```python
from build123d import *

# Parameters (mm, degrees)
SKETCH1_R                = 13
SKETCH1_R_2              = 11
BOSS_EXTRUDE1_DEPTH      = 10
BOSS_EXTRUDE2_REACH      = 32.741
BOSS_EXTRUDE2_END_RADIUS = 13
SKETCH2_W                = 10
SKETCH2_H                = 26
SKETCH2_3_R              = 13
BOSS_EXTRUDE3_DEPTH      = 10


with BuildPart() as part:
    # Sketch1 → Boss-Extrude1 (new body)
    with BuildSketch(Plane(origin=(0, 0, 0), x_dir=(0, 0, -1), z_dir=(1, 0, 0))):
        Circle(SKETCH1_R)
        Circle(SKETCH1_R_2, mode=Mode.SUBTRACT)
    extrude(amount=BOSS_EXTRUDE1_DEPTH)

    # Boss-Extrude2: up to this cylinder (the profile starts outside it)
    boss_extrude2_end = Plane(origin=(5, 0, 0), z_dir=(-1, 0, 0)) * Cylinder(BOSS_EXTRUDE2_END_RADIUS, 92.482, mode=Mode.PRIVATE)
    # Sketch2 → Boss-Extrude2 (add, up to the surface)
    with BuildSketch(Plane(origin=(0, 13, 0), x_dir=(1, 0, 0), z_dir=(0, 1, 0)), mode=Mode.PRIVATE) as boss_extrude2_sk1:
        with Locations((5, 0)):
            Rectangle(SKETCH2_W, SKETCH2_H)
    boss_extrude2_tool1 = extrude(boss_extrude2_sk1.sketch, amount=-BOSS_EXTRUDE2_REACH, mode=Mode.PRIVATE) - boss_extrude2_end
    add(boss_extrude2_tool1.solids().sort_by_distance((5, 13, 0))[0])
    add(boss_extrude2_tool1.solids().sort_by_distance((5, 13, 0))[1])

    # Sketch2_3 → Boss-Extrude3 (add)
    with BuildSketch(Plane(origin=(0, 13, 0), x_dir=(1, 0, 0), z_dir=(0, 1, 0))):
        with BuildLine():
            Line((10, -13), (10, 13))
            Line((10, 13), (-9.411981237, 13))
            ThreePointArc((-9.411981237, 13), (-15, 13.845319391), (-20.588018763, 13))
            Line((-20.588018763, 13), (-30, 13))
            Line((-30, 13), (-30, -13))
            Line((-30, -13), (-20.588018763, -13))
            ThreePointArc((-20.588018763, -13), (-15, -13.845319391), (-9.411981237, -13))
            Line((-9.411981237, -13), (10, -13))
        make_face()
        with Locations(Location((-15, 0, 0), (0, 0, 270))):
            Circle(SKETCH2_3_R, mode=Mode.SUBTRACT)
    extrude(amount=BOSS_EXTRUDE3_DEPTH)


solid = part.part
```
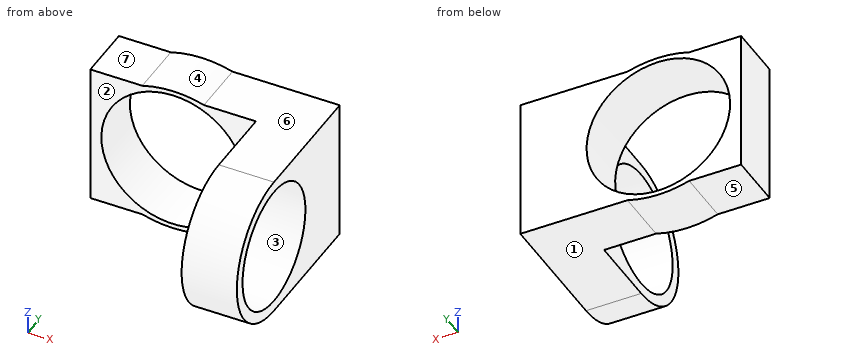
Part model, mm, in its own coordinate system. Face numbers are marked on the shaded views. A direction names the side the tool comes from. Round coordinates to 2 decimals unless told otherwise and drop trailing zeros. Write each loop counter-clockwise with the first axis right and the second up, starting at its lowest first coordinate (ties: lowest second). Pieces come first, ordered by that corner, then holes.
Item 1: Which spindle directions (+Z, -Z, +X, -X, +Y, -Y) get a long thin tool onto all of the face, cutting with end or side? Do the marked faces 4, 5, 6 and 7. Say none if no direction does.
Results:
face 4: +Z, +Y, -Y
face 5: -Z, -X, +Y, -Y
face 6: +Z, +X, +Y, -Y
face 7: +Z, -X, +Y, -Y
Item 2: Drop flat-ended pins along their axis: pin 1 Ø10 at (x, y) = (-25, 12) entering from -Z; pin 2 Ø8 at (x, y) = (-3.5, -7.5) entering from -Z; pin 3 Ø10.5 at (x, y) = (-26, 19.5) entering from +Z; pin 4 Ø2 at (y, z) = (3.5, 9.5) entering from +X. Give the stop position or say it passes through.
Results:
pin 1: stops at z = -13.14
pin 2: stops at z = -11.75
pin 3: stops at z = 13
pin 4: stops at x = 10
Item 3: Cut at C-C, the plane y = 19.5. Give the cut face in (x, z).
Results:
outline: (-30, -13) - (-20.59, -13) arc R18.89 ccw to (-9.41, -13) - (10, -13) - (10, 13) - (-9.41, 13) arc R18.89 ccw to (-20.59, 13) - (-30, 13) - close; hole circle Ø26 at (-15, 0)
Item 4: Probe L1, parallel to X at y = 18, z = 0; L2, parallel to Y at x = 5.25, z = 0; L3, parallel to Z at x = 5.5, y = -4.5. List the from-to ranges inside material, lowest first.
Results:
L1: x = -30 to -28, -2 to 10
L2: y = -13 to -11, 11 to 23
L3: z = -12.2 to -10.04, 10.04 to 12.2
Item 5: Cut at D-D, the plane x = 3.5. Give the cut face in (y, z), plus the area to 3 significant figures.
Results:
outline: (0, -13) - (23, -13) - (23, 13) - (0, 13) arc R13 ccw to start; hole circle Ø22 at (0, 0)
area: 483 mm2
Item 6: Two-plate mould, pull along Z, no slides. Class the marked faces 1, 2 and 3: +Z half, -Z half, draft (parallel to the pull), parting line (faces both ways), or undercut.
Results:
face 1: -Z half
face 2: draft
face 3: undercut
Item 7: Cut at A-A, the plane z = 0. Give the cut face in (x, y).
Results:
outline: (-30, 13) - (-28, 13) - (-28, 23) - (-30, 23) - close; (-2, 13) - (0, 13) - (0, 11) - (10, 11) - (10, 23) - (-2, 23) - close; (0, -13) - (10, -13) - (10, -11) - (0, -11) - close
Item 8: Cut at B-B, the plane x = -15. Give the cut face in (y, z).
Results:
outline: (13, -13.85) - (23, -13.85) - (23, -13) - (13, -13) - close; (13, 13) - (23, 13) - (23, 13.85) - (13, 13.85) - close
